The model under review builds one solid part; all positions refer to its coordinate system, in mm. Face numbers are marked on the shaded views. A direction names the side the tool comes from. Round coordinates to 2 decimals unless told otherwise and drop trailing zeros. Order: outer loops, then holes, each group sorted by start corner. A loop starts at its lowest first (then second) coordinate and runs counter-clockwise, first axis right, second up. Notation, with made-up numbers: (39.5, -0.75) - (61.5, -0.75) arc R8 cw to (61.5, 7.25) - close; hole circle Ø5 at (14, -29.5). An arc over 180 degrees is marked (long way). One line per question, with ' | ' between items. Start each with the question number.
Item 1: Tool access review of the marked faces 1 and 2: name each direction out of +Z, -Z, +X, -X, +Y, -Y from which nothing blocks a thin tool from reaching the whole face with its end or side.
Item 2: For L1, parallel to Z at x = 13, y = 11.5; L2, parallel to Y at x = 13, z = 23; L3, parallel to Y at x = 11.75, z = 1, list the stretches that pass through material, from the lowest coordinate up. Write a range as [from, to].
Item 3: Add section B-B on x = 11. State the section outline as (y, z) points.
Item 4: Add section A-A on x = 5. State the section outline as (y, z) points, and give its area (3 significant figures).
Item 5: Insertion check: pin 1 Ø2 at (y, z) = (-23.5, 8.5) entering from +X; pin 2 Ø2 at (x, y) = (4, -28) entering from -Z; pin 3 Ø1.5 at (x, y) = (9.5, -6) entering from -Z; pin 4 Ø3 at (y, z) = (-2, -10) entering from +X. Each pin has a flat end and moves straight along its axis. Give the tip position at first contact, or say it passes through.
from build123d import *

# Parameters (mm, degrees)
SKETCH1_W                = 15
SKETCH1_H                = 15
BOSS_EXTRUDE1_DEPTH      = 15
BOSS_EXTRUDE2_DEPTH      = 40
BOSS_EXTRUDE2_DEPTH_BACK = 12
SKETCH2_R                = 7.5


with BuildPart() as part:
    # Sketch1 → Boss-Extrude1 (new body)
    with BuildSketch(Plane(origin=(0, 0, 0), x_dir=(1, 0, 0), z_dir=(0, 1, 0))):
        with Locations((7.5, 7.5)):
            Rectangle(SKETCH1_W, SKETCH1_H)
    extrude(amount=BOSS_EXTRUDE1_DEPTH)

    # Sketch2 → Boss-Extrude2 (add, two sides: drawn at the far end of the back side and taken through both)
    with BuildSketch(Plane(origin=(0, 0, 0), x_dir=(1, 0, 0), z_dir=(0, -0.8191520442889992, 0.5735764363510355)).offset(-BOSS_EXTRUDE2_DEPTH_BACK)):
        with Locations(Location((7.5, 0, 0), (0, 0, 270))):
            Circle(SKETCH2_R)
    extrude(amount=BOSS_EXTRUDE2_DEPTH + BOSS_EXTRUDE2_DEPTH_BACK)


solid = part.part
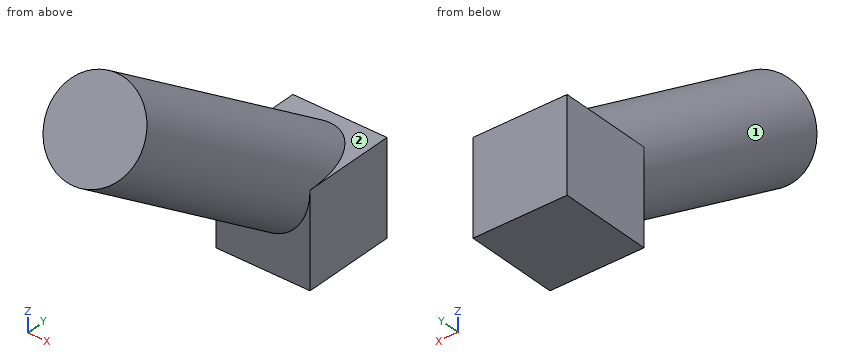
Determined:
1) face 1: none | face 2: +Z, +Y
2) L1: [-15, 0] | L2: [-32.73, -23.96] | L3: [-12.2, 9.35]
3) outline: (-36.57, 17.51) - (0, -8.1) - (0, -15) - (15, -15) - (15, 0) - (11.56, 0) - (-28.96, 28.38) - close
4) outline: (-36.82, 17.15) - (0, -8.63) - (0, -15) - (15, -15) - (15, 0) - (12.33, 0) - (-28.71, 28.74) - close | area: 844 mm2
5) pin 1: x = 12.58 | pin 2: z = 10.6 | pin 3: z = -5.2 | pin 4: through
